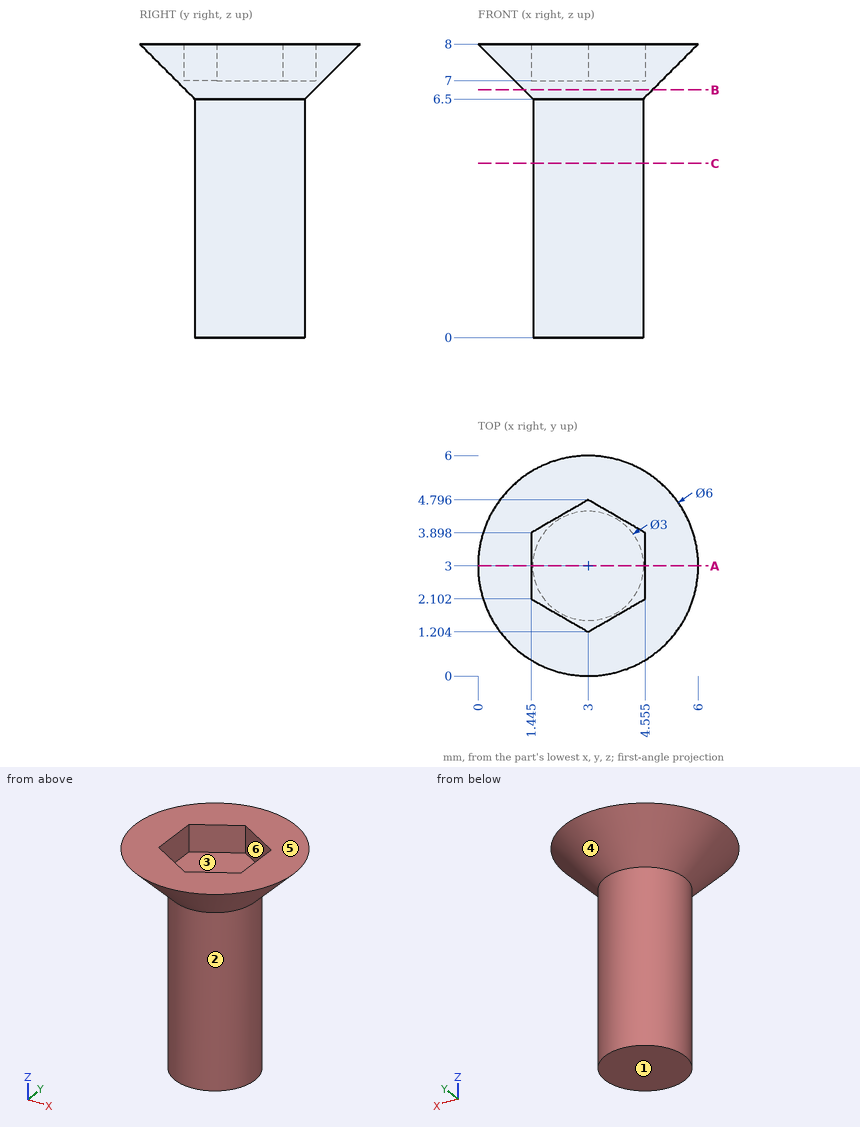
Print and shaded views of the part. All mm, measured from the part's lowest x, y and z. A direction names the side the tool comes from. Give positions to 0.01 mm unless a question says otherwise; leave off trailing zeros. Loops run counter-clockwise (first coordinate to the right, second up) from the corner with the lowest first, then second, coordinate; pieces in that order, holes last.
1) Flat gauge pins, fed straight in: pin 1 Ø0.8 at (y, z) = (3.5, 7.5) entering from +X; pin 2 Ø2 at (y, z) = (3, 2) entering from +X; pin 3 Ø3 at (x, z) = (3, 5.5) entering from +Y. Where does each tip first touch, or does it go through?
2) Tool access for the marked faces 1, 2 and 3: list every direction of +Z, -Z, +X, -X, +Y, -Y with a clear straight run to the whole face (end or side of a thin tool).
3) Wall check: line 1 (Z direction, x = 4.3, y = 3.2); line 2 (X direction, y = 1.3, z = 7.75) (1 decimal); line 3 (Y direction, x = 4.1, z = 1). Give the ranges that are in metal, low to high.
4) Saw through at B-B (z = 6.75). Write the cut outline in (x, y).
5) Saw through at A-A (y = 3). Write the cut outline in (x, z) (1 decimal).
6) Pull direction Y, two halves, no side cores. Call the marked faces 4, 5 and 6: +Y half, -Y half, draft (parallel to the pull), parting line (faces both ways), or undercut.
7) Saw through at C-C (z = 4.75). Write the cut outline in (x, y).
Answer block:
1. pin 1: stops at x = 5.86
1. pin 2: stops at x = 4.5
1. pin 3: stops at y = 5
2. face 1: -Z, +X, -X, +Y, -Y
2. face 2: -Z
2. face 3: +Z
3. line 1: z = 0 to 7
3. line 2: x = 0.8 to 2.8, 3.2 to 5.2
3. line 3: y = 1.98 to 4.02
4. outline: circle Ø3.5 at (3, 3)
5. outline: (0, 8) - (1.5, 6.5) - (1.5, 0) - (4.5, 0) - (4.5, 6.5) - (6, 8) - (4.6, 8) - (4.6, 7) - (1.4, 7) - (1.4, 8) - close
6. face 4: parting line
6. face 5: draft
6. face 6: undercut
7. outline: circle Ø3 at (3, 3)
